Job drawing, mm, ordinate dimensions from the low corner. One solid piece. A direction names the side the tool comes from. Give positions to 0.01 mm unless a question says otherwise; leave off trailing zeros. Loops run counter-clockwise (first coordinate to the right, second up) from the corner with the lowest first, then second, coordinate; pieces in that order, holes last. Notation, with made-up numbers: (62.25, 84) - (116.25, 84) arc R34 cw to (116.25, 117) - close; hole circle Ø5 at (38, 18.25). An arc over 180 degrees is marked (long way). Answer as CSV lines item,"result". Start each with the question number.
Item 1: Pull direction X, two halves, no side cores. Call the marked faces 6, 7 and 8: pulls with the +X half, pulls with the -X half, needs draft (parallel to the pull), parting line crosses it, or undercut.
Item 2: Drill centre lines: L1, parallel to X at y = 2.5, z = 22; L2, parallel to X at y = 12, z = 8; L3, parallel to X at y = 27.5, z = 2 (1 decimal). Where is each one in solid material? Low to high. Write a range as from..to.
Item 3: Saw through at B-B on y = 7.5. Give the cut face in (x, z).
Item 4: Pin check, flat tips, straight feed: pin 1 (9.5 mm diameter, centred on y = 9.5, z = 17.5, fed in from -X); pin 2 (5.5 mm diameter, centred on y = 11, z = 15.5, fed in from +X); pin 3 (8.5 mm diameter, centred on x = 29.5, z = 16.5, fed in from -Y) (1 decimal); pin 4 (17.5 mm diameter, centred on x = 57.5, y = 17, fed in from +Z). Stop position of each tip, or through.
Item 5: Saw through at D-D on y = 14. Give the cut face in (x, z).
Item 6: Tool access for the marked faces 1, 2, 3, 4 and 5: list every direction of +Z, -Z, +X, -X, +Y, -Y with a clear straight run to the whole face (end or side of a thin tool).
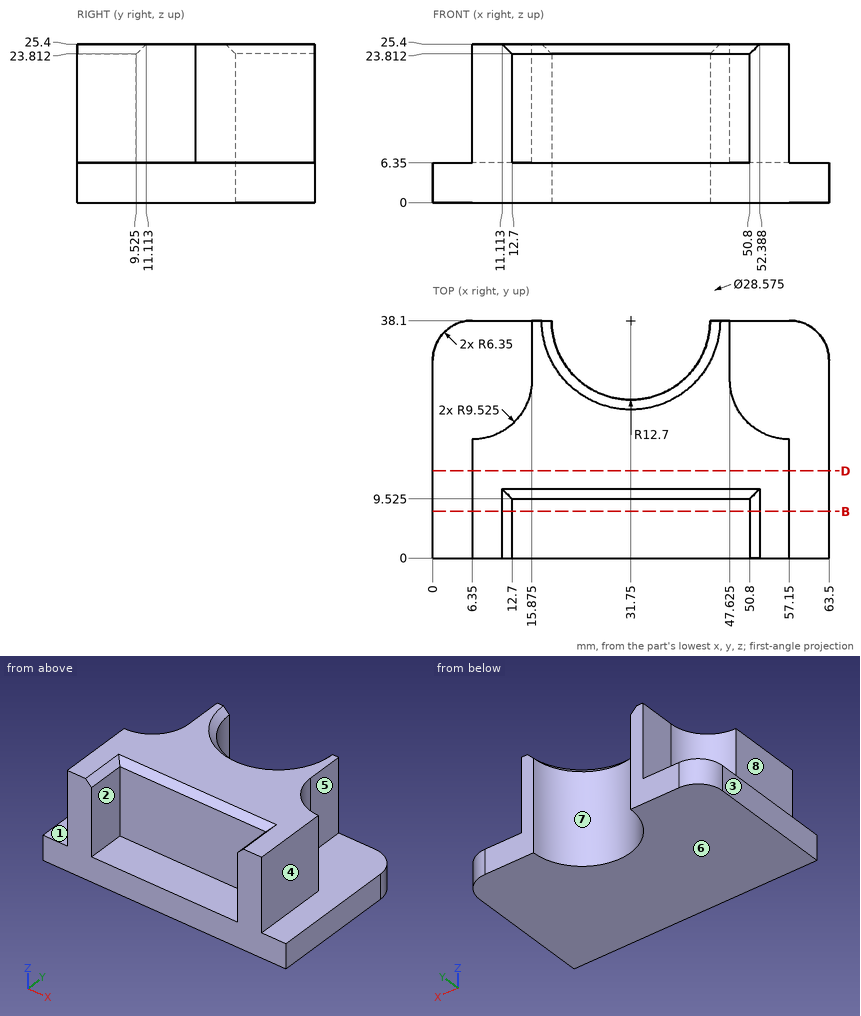
Responses:
1,face 6,"needs draft"
1,face 7,"undercut"
1,face 8,"pulls with the -X half"
2,L1,"6.35..12.7, 50.8..57.15"
2,L2,"6.35..57.15"
2,L3,"0..24.8, 38.7..63.5"
3,outline,"(0, 0) - (63.5, 0) - (63.5, 6.35) - (57.15, 6.35) - (57.15, 25.4) - (52.39, 25.4) - (50.8, 23.81) - (50.8, 6.35) - (12.7, 6.35) - (12.7, 23.81) - (11.11, 25.4) - (6.35, 25.4) - (6.35, 6.35) - (0, 6.35) - close"
4,pin 1,"x = 6.35"
4,pin 2,"x = 57.15"
4,pin 3,"y = 9.5"
4,pin 4,"z = 25.4"
5,outline,"(0, 0) - (63.5, 0) - (63.5, 6.35) - (57.15, 6.35) - (57.15, 25.4) - (6.35, 25.4) - (6.35, 6.35) - (0, 6.35) - close"
6,face 1,"+Z, -X, +Y"
6,face 2,"+Z, -Y"
6,face 3,"+Z, -Z, -X, +Y, -Y"
6,face 4,"+Z, +X, +Y, -Y"
6,face 5,"+Z, +X, +Y"
